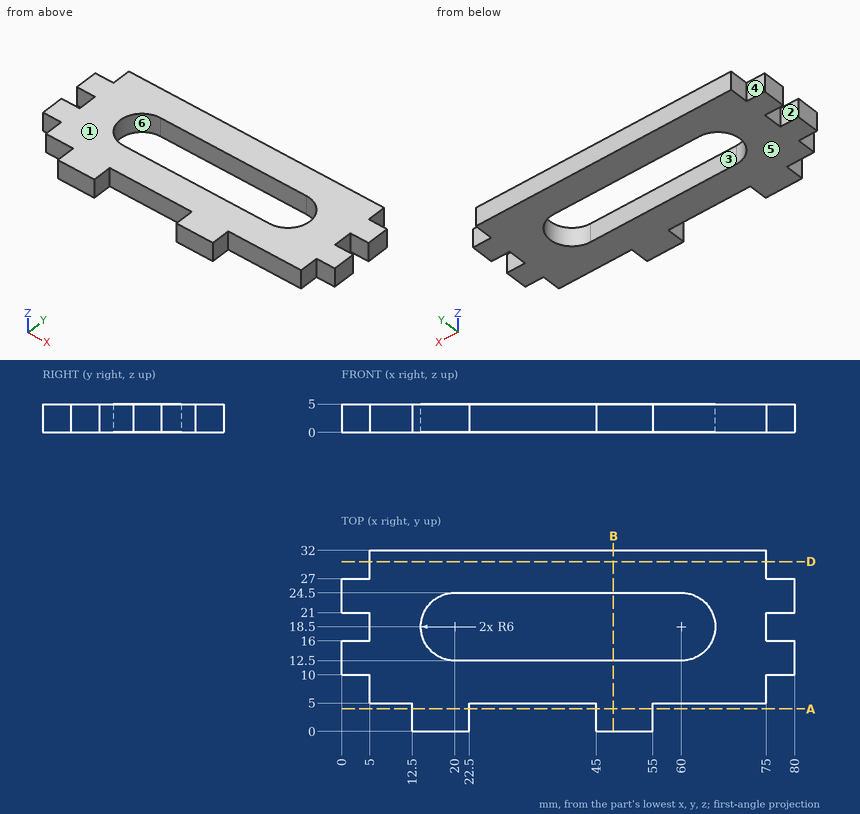
The figure shows three views and two pictorial views of one solid part (mm, origin at its lowest corner). Answer the questions. A direction names the side the tool comes from. Coordinates: 2 decimals unless noted, no trailing zeros. Order: outer loops, then holes, each group sorted by start corner. A loop starts at its lowest first (then second) coordinate and runs counter-clockwise, first axis right, second up.
Q1. A cutting plane is placed at B-B, the plane x = 48. Write down the section's boundary in (y, z), and give its area (3 significant figures).
Q2. A cutting plane is placed at A-A, the plane y = 4. Write down the section's boundary in (x, z), and give its area (3 significant figures).
Q3. Which of the six approach directions +Z, -Z, +X, -X, +Y, -Y give full straight-line access (tool end or side, diameter ignored) to the marked faces 1, 2 and 3?
Q4. Consider line 1 (Y direction, x = 59, z = 1.8); line 2 (Y direction, x = 46.5, z = 2.15); line 3 (X direction, y = 4.5, z = 2.45). Determine where each line is inside the solid, lowest interval first.
Q5. Given P1, Ø2.5, axis at y = 2, z = 1.5, coming from the -X side; P2, Ø1.5, axis at y = 29, z = 2.5, coming from the -X side; P3, Ø1.5, axis at x = 77, z = 2, coming from the +Y side; P4, Ø6, axis at x = 25.5, y = 24.5, coming from the -Z side, each flat-ended and moving along its own axis, determine where each tip first touches the part or whether it passes through.
Q6. A cutting plane is placed at D-D, the plane y = 30. Write down the section's boundary in (x, z).
Q7. For a pull along Y with two mould halves and no side action, classify the marked faces 4, 5 and 6 as pulls with the +Y half, pulls with the -Y half, needs draft (parallel to the pull), parting line crosses it, or undercut.
Answers follow:
1. outline: (0, 0) - (12.5, 0) - (12.5, 5) - (0, 5) - close; (24.5, 0) - (32, 0) - (32, 5) - (24.5, 5) - close
1. area: 100 mm2
2. outline: (12.5, 0) - (22.5, 0) - (22.5, 5) - (12.5, 5) - close; (45, 0) - (55, 0) - (55, 5) - (45, 5) - close
2. area: 100 mm2
3. face 1: +Z, +X, -X, +Y, -Y
3. face 2: +Z, -Z, -X
3. face 3: +Z, -Z
4. line 1: y = 5 to 12.5, 24.5 to 32
4. line 2: y = 0 to 12.5, 24.5 to 32
4. line 3: x = 12.5 to 22.5, 45 to 55
5. P1: stops at x = 12.5
5. P2: stops at x = 5
5. P3: stops at y = 27
5. P4: stops at z = 0
6. outline: (5, 0) - (75, 0) - (75, 5) - (5, 5) - close
7. face 4: pulls with the +Y half
7. face 5: needs draft
7. face 6: undercut
